For this review, use the dimensioned drawing (mm, ordinates from the lowest corner) and the shaded views. Coordinates: 2 decimals unless noted, no trailing zeros. Loops run counter-clockwise (first coordinate to the right, second up) from the corner with the lowest first, then second, coordinate; pieces in that order, holes last. Notation, with made-up numbers: M 16.5,-11 L 45.5,-11 A17 ccw 45.5,15 Z; hole C 31.25,2.5 d8. An arc over 180 degrees is marked long. Write item = value, one per line. Start each with the question number.
Q1. Wall thickness on probe 1 along Y at (x, z) = (6.35, 1.5) (3 decimals); probe 2 along Y at (x, z) = (3.5, 2.85); probe 3 along X at (y, z) = (50.8, 2.35) (3 decimals): over which ranges is each line inside the solid? List them lowest first.
Q2. We need section B-B on x = 6.35. Give the boundary of the cut face in (y, z) (3 decimals), and give its area (3 significant figures).
Q3. We need section A-A on y = 50.8. Give the boundary of the cut face in (x, z) (3 decimals), and give its area (3 significant figures).
Q4. We need section C-C on z = 2.25. Give the boundary of the cut face in (x, y) (3 decimals).
Q5. Clearance check with flat-ended pins moving along their axes: pin 1 Ø5.5 at (x, y) = (6.35, 201.93) entering from +Z; pin 2 Ø5 at (x, y) = (2, 68) entering from -Z. State where each tip first meets the part, or that it passes through.
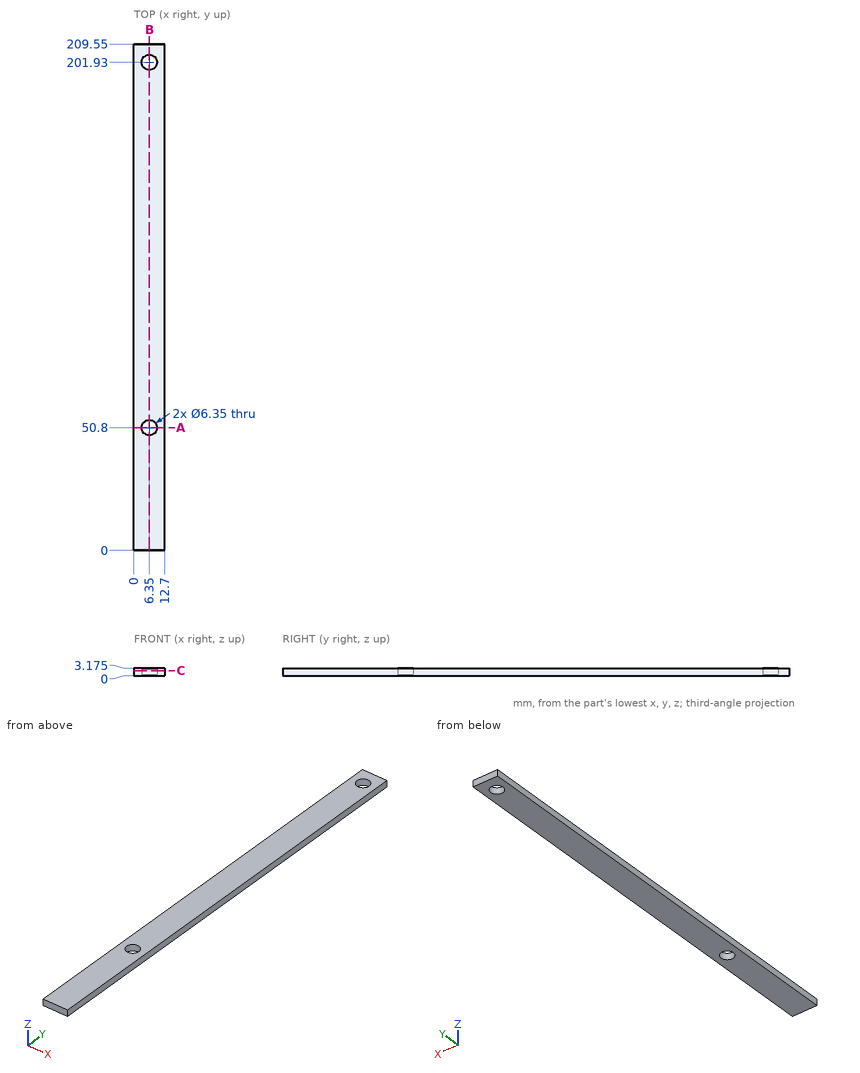
Returned:
q1.probe_1 = 0 to 47.625, 53.975 to 198.755, 205.105 to 209.55
q1.probe_2 = 0 to 49.4, 52.2 to 200.53, 203.33 to 209.55
q1.probe_3 = 0 to 3.175, 9.525 to 12.7
q2.outline = M 0,0 L 47.625,0 L 47.625,3.175 L 0,3.175 Z; M 53.975,0 L 198.755,0 L 198.755,3.175 L 53.975,3.175 Z; M 205.105,0 L 209.55,0 L 209.55,3.175 L 205.105,3.175 Z
q2.area = 625 mm^2
q3.outline = M 0,0 L 3.175,0 L 3.175,3.175 L 0,3.175 Z; M 9.525,0 L 12.7,0 L 12.7,3.175 L 9.525,3.175 Z
q3.area = 20.2 mm^2
q4.outline = M 0,0 L 12.7,0 L 12.7,209.55 L 0,209.55 Z; hole C 6.35,50.8 d6.35; hole C 6.35,201.93 d6.35
q5.pin_1 = through
q5.pin_2 = 0
